Verification items for the finished model (mm, model axes). Round coordinates to 2 decimals unless told otherwise and drop trailing zeros. Write each loop counter-clockwise with the first axis right and the second up, starting at its lowest first coordinate (ties: lowest second). Pieces come first, ordered by that corner, then holes. Notation, with made-up numbers: (69, 62) -> (106, 62) arc R14 cw to (106, 66) -> close; hole circle Ø10 at (74.25, 30.5). An arc over 180 degrees is marked (long way). Use CSV: the item, a comma, the result in double quotes.
```python
from build123d import *

# Parameters (mm, degrees)
F0_W     = 500
F0_H     = 700
F0_W_2   = 400
F0_H_2   = 450
F1_DEPTH = 2
F2_W     = 400
F2_H     = 130
F3_DEPTH = 4


with BuildPart() as f1:
    # F0 (on Front) → F1 (new body)
    with BuildSketch(Plane.XZ):
        Rectangle(F0_W, F0_H)
        with Locations((0, 75)):
            Rectangle(F0_W_2, F0_H_2, mode=Mode.SUBTRACT)
    extrude(amount=F1_DEPTH)

    # F2 (on face) → F3 (cut)
    with BuildSketch(Plane.XZ.offset(2)):
        with Locations((0, -255)):
            Rectangle(F2_W, F2_H)
    extrude(amount=-F3_DEPTH, mode=Mode.SUBTRACT)


solid = f1.part
```
Q1. Section check B-B (z = 211). Record the cut outline in (x, y).
Filled in:
outline,"(-250, -2) -> (-200, -2) -> (-200, 0) -> (-250, 0) -> close; (200, -2) -> (250, -2) -> (250, 0) -> (200, 0) -> close"
Q2. Section check C-C (y = -1.25). Record the cut outline in (x, z), plus the area to 3 significant figures.
Filled in:
outline,"(-250, -350) -> (250, -350) -> (250, 350) -> (-250, 350) -> close; hole (-200, -320) -> (200, -320) -> (200, -190) -> (-200, -190) -> close; hole (-200, -150) -> (200, -150) -> (200, 300) -> (-200, 300) -> close"
area,"118,000 mm²"
Q3. Section check A-A (x = 119.5). Record the cut outline in (y, z), plus the area to 3 significant figures.
Filled in:
outline,"(-2, -350) -> (0, -350) -> (0, -320) -> (-2, -320) -> close; (-2, -190) -> (0, -190) -> (0, -150) -> (-2, -150) -> close; (-2, 300) -> (0, 300) -> (0, 350) -> (-2, 350) -> close"
area,"240 mm²"
Q4. Material ranges on L1, parallel to Z at x = 29, y = -1.1; L2, parallel to X at y = -1.05, z = 150.5, recorded low to high.
Filled in:
L1,"-350 to -320, -190 to -150, 300 to 350"
L2,"-250 to -200, 200 to 250"
